CAD build for the part. Positions are in the model's coordinates, mm. A direction names the side the tool comes from. Coordinates: 2 decimals unless noted, no trailing zeros. Order: outer loops, then holes, each group sorted by start corner. A loop starts at its lowest first (then second) coordinate and runs counter-clockwise, first axis right, second up. Notation, with made-up numbers: M -20,87 L 30,87 A13 ccw 30,105 Z; hole C 26.25,-11 d5. An arc over 180 degrees is marked long. Write item = value, one per line.
from build123d import *

# Parameters (mm, degrees)
SKETCH_1_W          = 12
SKETCH_1_H          = 23
EXTRUDE_1_DEPTH     = 21
SKETCH_2_W          = 12
SKETCH_2_H          = 4
EXTRUDE_2_DEPTH     = 2
SKETCH_3_R          = 1
CUT_EXTRUDE_2_DEPTH = 2
SKETCH_4_R          = 1
CUT_EXTRUDE_3_DEPTH = 2
EXTRUDE_3_DEPTH     = 4
SKETCH_6_R          = 2
EXTRUDE_4_DEPTH     = 3
CUT_EXTRUDE_4_DEPTH = 29.727164844


with BuildPart() as part:
    # 草图1 → 凸台-拉伸1 (new body)
    with BuildSketch(Plane(origin=(0, 0, 0), x_dir=(1, 0, 0), z_dir=(0, 1, 0))):
        Rectangle(SKETCH_1_W, SKETCH_1_H)
    extrude(amount=EXTRUDE_1_DEPTH)

    # 草图2 → 凸台-拉伸2 (add)
    with BuildSketch(Plane(origin=(0, 5, 0), x_dir=(-1, 0, 0), z_dir=(0, -1, 0))):
        with Locations((0, -13.5)):
            Rectangle(SKETCH_2_W, SKETCH_2_H)
        with Locations((0, 13.5)):
            Rectangle(SKETCH_2_W, SKETCH_2_H)
    extrude(amount=EXTRUDE_2_DEPTH)

    # 草图3 → 切除-拉伸2 (cut)
    with BuildSketch(Plane(origin=(0, 5, 0), x_dir=(1, 0, 0), z_dir=(0, 1, 0))):
        with Locations(Location((0, -13.5, 0), (0, 0, 270))):
            Circle(SKETCH_3_R)
    extrude(amount=-CUT_EXTRUDE_2_DEPTH, mode=Mode.SUBTRACT)

    # 草图4 → 切除-拉伸3 (cut)
    with BuildSketch(Plane(origin=(0, 5, 0), x_dir=(1, 0, 0), z_dir=(0, 1, 0))):
        with Locations(Location((0, 13.5, 0), (0, 0, 270))):
            Circle(SKETCH_4_R)
    extrude(amount=-CUT_EXTRUDE_3_DEPTH, mode=Mode.SUBTRACT)

    # 草图5 → 凸台-拉伸3 (add)
    with BuildSketch(Plane.XZ):
        with BuildLine():
            ThreePointArc((6, 5.5), (4.242640687, 9.742640687), (0, 11.5))
            Line((0, 11.5), (0, 2))
            ThreePointArc((0, 2), (1.655410709, 1.501922338), (2.761139354, 0.173076923))
            ThreePointArc((2.761139354, 0.173076923), (5.126735615, 2.382856767), (6, 5.5))
        make_face()
        with BuildLine():
            Line((0, 2), (0, 11.5))
            ThreePointArc((0, 11.5), (-4.242640687, 9.742640687), (-6, 5.5))
            ThreePointArc((-6, 5.5), (-5.126735615, 2.382856767), (-2.761139354, 0.173076923))
            ThreePointArc((-2.761139354, 0.173076923), (-1.655410709, 1.501922338), (0, 2))
        make_face()
        with BuildLine():
            ThreePointArc((2.761139354, 0.173076923), (1.655410709, 1.501922338), (0, 2))
            Line((0, 2), (0, -0.5))
            ThreePointArc((0, -0.5), (1.4209964, -0.329302637), (2.761139354, 0.173076923))
        make_face()
        with BuildLine():
            Line((0, -0.5), (0, 2))
            ThreePointArc((0, 2), (-1.655410709, 1.501922338), (-2.761139354, 0.173076923))
            ThreePointArc((-2.761139354, 0.173076923), (-1.4209964, -0.329302637), (0, -0.5))
        make_face()
        with BuildLine():
            ThreePointArc((2.761139354, 0.173076923), (1.4209964, -0.329302637), (0, -0.5))
            Line((0, -0.5), (0, -4))
            ThreePointArc((0, -4), (2.121320344, -3.121320344), (3, -1))
            ThreePointArc((3, -1), (2.939678389, -0.401425887), (2.761139354, 0.173076923))
        make_face()
        with BuildLine():
            Line((0, -4), (0, -0.5))
            ThreePointArc((0, -0.5), (-1.4209964, -0.329302637), (-2.761139354, 0.173076923))
            ThreePointArc((-2.761139354, 0.173076923), (-2.501922338, -2.655410709), (0, -4))
        make_face()
        with BuildLine():
            ThreePointArc((6, 5.5), (4.242640687, 9.742640687), (0, 11.5))
            Line((0, 11.5), (0, 2))
            ThreePointArc((0, 2), (1.655410709, 1.501922338), (2.761139354, 0.173076923))
            ThreePointArc((2.761139354, 0.173076923), (5.126735615, 2.382856767), (6, 5.5))
        make_face()
        with BuildLine():
            Line((0, 2), (0, 11.5))
            ThreePointArc((0, 11.5), (-4.242640687, 9.742640687), (-6, 5.5))
            ThreePointArc((-6, 5.5), (-5.126735615, 2.382856767), (-2.761139354, 0.173076923))
            ThreePointArc((-2.761139354, 0.173076923), (-1.655410709, 1.501922338), (0, 2))
        make_face()
        with BuildLine():
            ThreePointArc((2.761139354, 0.173076923), (1.655410709, 1.501922338), (0, 2))
            Line((0, 2), (0, -0.5))
            ThreePointArc((0, -0.5), (1.4209964, -0.329302637), (2.761139354, 0.173076923))
        make_face()
        with BuildLine():
            Line((0, -0.5), (0, 2))
            ThreePointArc((0, 2), (-1.655410709, 1.501922338), (-2.761139354, 0.173076923))
            ThreePointArc((-2.761139354, 0.173076923), (-1.4209964, -0.329302637), (0, -0.5))
        make_face()
        with BuildLine():
            ThreePointArc((2.761139354, 0.173076923), (1.4209964, -0.329302637), (0, -0.5))
            Line((0, -0.5), (0, -4))
            ThreePointArc((0, -4), (2.121320344, -3.121320344), (3, -1))
            ThreePointArc((3, -1), (2.939678389, -0.401425887), (2.761139354, 0.173076923))
        make_face()
        with BuildLine():
            Line((0, -4), (0, -0.5))
            ThreePointArc((0, -0.5), (-1.4209964, -0.329302637), (-2.761139354, 0.173076923))
            ThreePointArc((-2.761139354, 0.173076923), (-2.501922338, -2.655410709), (0, -4))
        make_face()
        with BuildLine():
            ThreePointArc((6, 5.5), (4.242640687, 9.742640687), (0, 11.5))
            Line((0, 11.5), (0, 2))
            ThreePointArc((0, 2), (1.655410709, 1.501922338), (2.761139354, 0.173076923))
            ThreePointArc((2.761139354, 0.173076923), (5.126735615, 2.382856767), (6, 5.5))
        make_face()
        with BuildLine():
            Line((0, 2), (0, 11.5))
            ThreePointArc((0, 11.5), (-4.242640687, 9.742640687), (-6, 5.5))
            ThreePointArc((-6, 5.5), (-5.126735615, 2.382856767), (-2.761139354, 0.173076923))
            ThreePointArc((-2.761139354, 0.173076923), (-1.655410709, 1.501922338), (0, 2))
        make_face()
        with BuildLine():
            ThreePointArc((2.761139354, 0.173076923), (1.655410709, 1.501922338), (0, 2))
            Line((0, 2), (0, -0.5))
            ThreePointArc((0, -0.5), (1.4209964, -0.329302637), (2.761139354, 0.173076923))
        make_face()
        with BuildLine():
            Line((0, -0.5), (0, 2))
            ThreePointArc((0, 2), (-1.655410709, 1.501922338), (-2.761139354, 0.173076923))
            ThreePointArc((-2.761139354, 0.173076923), (-1.4209964, -0.329302637), (0, -0.5))
        make_face()
        with BuildLine():
            ThreePointArc((2.761139354, 0.173076923), (1.4209964, -0.329302637), (0, -0.5))
            Line((0, -0.5), (0, -4))
            ThreePointArc((0, -4), (2.121320344, -3.121320344), (3, -1))
            ThreePointArc((3, -1), (2.939678389, -0.401425887), (2.761139354, 0.173076923))
        make_face()
        with BuildLine():
            Line((0, -4), (0, -0.5))
            ThreePointArc((0, -0.5), (-1.4209964, -0.329302637), (-2.761139354, 0.173076923))
            ThreePointArc((-2.761139354, 0.173076923), (-2.501922338, -2.655410709), (0, -4))
        make_face()
    extrude(amount=EXTRUDE_3_DEPTH)

    # 草图6 → 凸台-拉伸4 (add)
    with BuildSketch(Plane.XZ.offset(4)):
        with Locations(Location((0, 5.5, 0), (0, 0, 270))):
            Circle(SKETCH_6_R)
    extrude(amount=EXTRUDE_4_DEPTH)

    # 草图7 → 切除-拉伸4 (cut, through all)
    with BuildSketch(Plane(origin=(6, 0, 0), x_dir=(0, 0, -1), z_dir=(1, 0, 0))):
        Polygon((-11.5, 21), (-11.5, 19), (-7.5, 21), align=None)
    extrude(amount=-CUT_EXTRUDE_4_DEPTH, mode=Mode.SUBTRACT)


solid = part.part
(1) Pin check, flat tips, straight feed: pin 1 Ø1.8 at (x, z) = (3.5, 10) entering from -Y; pin 2 Ø0.9 at (x, y) = (3, 1) entering from +Z; pin 3 Ø6 at (x, y) = (-2.5, 12.5) entering from -Z; pin 4 Ø1.2 at (x, z) = (0, 13.5) entering from +Y. Stop position of each tip, or through.
Evaluation:
pin_1 = -4
pin_2 = 11.5
pin_3 = -11.5
pin_4 = through
(2) Slice it at B-B, the plane y = -2. Write the cut outline in (x, z).
Evaluation:
outline = M -2.76,0.17 A3 ccw long 2.76,0.17 A6 ccw long Z
(3) Slice it at C-C, the plane x = -3.75. Write the cut outline in (y, z).
Evaluation:
outline = M -4,0.82 L 0,0.82 L 0,-11.5 L 3,-11.5 L 3,-15.5 L 5,-15.5 L 5,-11.5 L 21,-11.5 L 21,7.5 L 19,11.5 L 5,11.5 L 5,15.5 L 3,15.5 L 3,11.5 L 0,11.5 L 0,10.18 L -4,10.18 Z
(4) Tool access for faces 4 (the face through (0, 3, 15)), 5 (the face through (-1.2, -5.5, 7.1)), 6 (the face through (-5, 0, 10)), 7 (the face through (5, 0, 10)), 8 (the face through (0, 12, 11.5)): list every direction of +Z, -Z, +X, -X, +Y, -Y with a clear straight run to the whole face (end or side of a thin tool).
Evaluation:
face_4 = +Z, +X, -X, -Y
face_5 = -Y
face_6 = +Z, -X, -Y
face_7 = +Z, +X, -Y
face_8 = +Z, +X, -X, +Y
(5) Pull direction Z, two halves, no side cores. Call faces 1 (the face through (0, 1, 11.5)), 2 (the face through (-0.383, 4.014, -12.576)), 3 (the face through (0, 5, -12)): +Z half, -Z half, draft (parallel to the pull), parting line (faces both ways), or undercut.
Evaluation:
face_1 = +Z half
face_2 = undercut
face_3 = draft
(6) Slice it at D-D, the plane z = -13. Write the cut outline in (x, y).
Evaluation:
outline = M -6,3 L -0.87,3 L -0.87,5 L -6,5 Z; M 0.87,3 L 6,3 L 6,5 L 0.87,5 Z
(7) Wall check: line 1 (X direction, y = 4.5, z = -13.5); line 2 (Z direction, x = 2.25, y = 10); line 3 (Y direction, x = 5.75, z = 5). Give the ranges that are in metal, low to high. Write a range as from..to.
Evaluation:
line_1 = -6..-1, 1..6
line_2 = -11.5..11.5
line_3 = -4..21
(8) Slice it at A-A, the plane z = 13.5. Write the cut outline in (x, y).
Evaluation:
outline = M -6,3 L -1,3 L -1,5 L -6,5 Z; M 1,3 L 6,3 L 6,5 L 1,5 Z
